```python
from build123d import *

# Parameters (mm, degrees)
FILLET1_SIZE  = 0.5
CHAMFER1_SIZE = 0.4


with BuildPart() as part:
    # Sketch1 → Revolve1 (revolve)
    with BuildSketch(Plane.XY, mode=Mode.PRIVATE) as revolve1_sk:
        Polygon((10, 0), (10, 10), (0, 10), (0, 9), (9, 9), (9, 0), align=None)
    revolve(revolve1_sk.sketch.rotate(Axis((0, 10, 0), (0, -1, 0)), 180), axis=Axis((0, 10, 0), (0, -1, 0)))

    # Fillet1
    # a fillet whose section is not a circle: 0.5 mm, written as the material it takes off along each edge
    with BuildSketch(Plane(origin=(0, 10, 0), x_dir=(-1, 0, 0), z_dir=(0, 0, 1))) as fillet1_piece_1:
        with BuildLine():
            add(Edge.make_bspline([(10, FILLET1_SIZE), (10, FILLET1_SIZE * 0.831801948466), (10, FILLET1_SIZE * 0.663603896932), (10 - FILLET1_SIZE * 0.0716919198361, FILLET1_SIZE * 0.292893218813), (10 - FILLET1_SIZE * 0.292893218813, FILLET1_SIZE * 0.0716919198361), (10 - FILLET1_SIZE * 0.663603896932, 0), (10 - FILLET1_SIZE * 0.831801948466, 0), (10 - FILLET1_SIZE, 0)], knots=[0, 0, 0, 0, 0, 0, 0.5, 0.5, 1, 1, 1, 1, 1, 1], degree=5))
            Line((10 - FILLET1_SIZE, 0), (10, 0))
            Line((10, 0), (10, FILLET1_SIZE))
        make_face()
    revolve(axis=Axis((0, 10, 0), (0, -1, 0)), mode=Mode.SUBTRACT)

    # Chamfer1
    chamfer1_edges = [part.edges().sort_by_distance(p)[0] for p in [
        (10, 0, 0),
    ]]
    chamfer(chamfer1_edges, length=CHAMFER1_SIZE)


solid = part.part
```
Geometry check sheet. Reference: the model listing, model coordinates, mm. A direction names the side the tool comes from. Coordinates: 2 decimals unless noted, no trailing zeros. Loops run counter-clockwise (first coordinate to the right, second up) from the corner with the lowest first, then second, coordinate; pieces in that order, holes last.
Item 1: Thickness scan on line 1 (Z direction, x = 0, y = 2.75); line 2 (Y direction, x = -0.25, z = -8.5); line 3 (Z direction, x = -3, y = 6.25). Record the ranges inside material, lowest first.
Item 2: Access from +Z, -Z, +X, -X, +Y, -Y to the whole of each face (thin tool, end or side, straight path). Record for faces 1 (the face through (6.633, 4.437, -6.083)), 2 (the face through (0, 10, 0)).
Item 3: Sectioned sample at A-A, the plane y = 2.5. Record the boundary of the cut face in (x, z), then the cut area to 3 significant figures.
Item 4: Release check for a two-part mould opening along Z. For faces 3 (the face through (6, 0, 7)), 4 (the face through (0, 9, 0)), 5 (the face through (10, 5, 0)) record: released by +Z, released by -Z, zero draft, split by the parting line, or undercut.
Item 5: Go/stop test with flat-tipped pins: pin 1 Ø2 at (y, z) = (8, 3) entering from +X; pin 2 Ø1 at (y, z) = (3.5, -6) entering from +X; pin 3 Ø2 at (x, z) = (-2.5, -3.5) entering from -Y. Record where each tip stops, or that it passes through.
Check result:
1. line 1: z = -10 to -9, 9 to 10
1. line 2: y = 9 to 10
1. line 3: z = -9.54 to -8.49, 8.49 to 9.54
2. face 1: -Y
2. face 2: +Z, -Z, +X, -X, +Y
3. outline: circle Ø20 at (0, 0); hole circle Ø18 at (0, 0)
3. area: 59.7 mm2
4. face 3: zero draft
4. face 4: undercut
4. face 5: split by the parting line
5. pin 1: stops at x = 9.8
5. pin 2: stops at x = 8.35
5. pin 3: stops at y = 9
